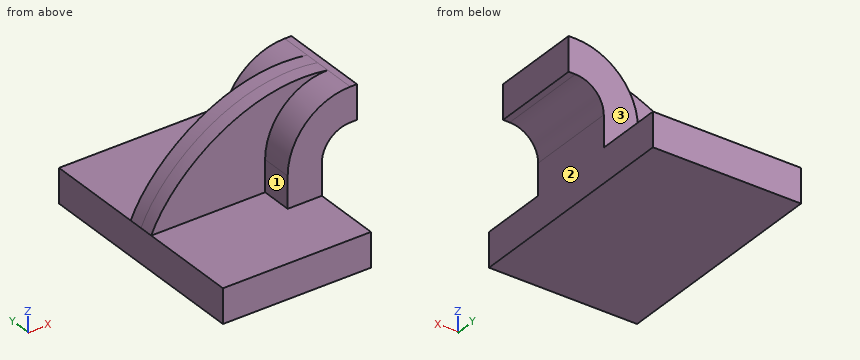
```python
from build123d import *

# Parameters (mm, degrees)
F1_DEPTH = 63.5
F2_DEPTH = 25.4
F3_DEPTH = 7.9375


with BuildPart() as f1:
    # F0 (on Front) → F1 (new body, symmetric)
    with BuildSketch(Plane.XZ):
        Polygon((-41.275, 9.525), (-41.275, -9.525), (41.275, -9.525), (41.275, 9.525), (22.225, 9.525), align=None)
    extrude(amount=F1_DEPTH, both=True)

    # F0 (on Front) → F2 (join, symmetric)
    with BuildSketch(Plane.XZ):
        with BuildLine():
            Line((22.225, 9.525), (41.275, 9.525))
            Line((41.275, 9.525), (41.275, 27.0002))
            ThreePointArc((41.275, 27.0002), (45.9246798487, 38.2255201513), (57.15, 42.8752))
            Line((57.15, 42.8752), (60.8642640084, 42.8752))
            Line((60.8642640084, 42.8752), (60.8642640084, 61.9252))
            Line((60.8642640084, 61.9252), (57.15, 61.9252))
            ThreePointArc((57.15, 61.9252), (32.4542956671, 51.6959043329), (22.225, 27.0002))
            Line((22.225, 27.0002), (22.225, 9.525))
        make_face()
    extrude(amount=F2_DEPTH, both=True)

    # F0 (on Front) → F3 (join, symmetric)
    with BuildSketch(Plane.XZ):
        with BuildLine():
            add(Edge.make_bspline(
                [(-41.275, 9.525), (-30.5388011038, 34.9970385432), (9.5851859078, 69.7711631656), (57.15, 61.9252)],
                knots=[0, 0, 0, 0, 111.5045361635, 111.5045361635, 111.5045361635, 111.5045361635], degree=3))
            Line((-41.275, 9.525), (22.225, 9.525))
            Line((22.225, 9.525), (22.225, 27.0002))
            ThreePointArc((22.225, 27.0002), (32.4542956671, 51.6959043329), (57.15, 61.9252))
        make_face()
    extrude(amount=F3_DEPTH, both=True)


solid = f1.part
```
CAD build for the part. Positions are in the model's coordinates, mm. Face numbers are marked on the shaded views. A direction names the side the tool comes from. Give positions to 0.01 mm unless a question says otherwise; leave off trailing zeros. Order: outer loops, then holes, each group sorted by start corner. A loop starts at its lowest first (then second) coordinate and runs counter-clockwise, first axis right, second up. Notation, with made-up numbers: M 53.25,67.25 L 103.25,67.25 A21 cw 103.25,94.25 Z; hole C 30,43 d7. An arc over 180 degrees is marked long. Put each result on its own line as item: value. Start each with the question number.
(1) Which spindle directions (+Z, -Z, +X, -X, +Y, -Y) get a long thin tool onto all of the face, cutting with end or side? Do the marked faces 1, 2 and 3. Say none if no direction does.
(2) Flat gauge pins, fed straight in: pin 1 Ø1.9 at (x, y) = (59, -9.5) entering from -Z; pin 2 Ø1.9 at (x, y) = (59, -9.5) entering from +Z; pin 3 Ø5 at (y, z) = (14, 19) entering from +X (3 decimals). Where does each tip first touch, or does it go through?
(3) Drill centre lines: line 1 along Y through (x, z) = (-25, 14.5); line 2 along Z through (x, y) = (-31, 27.5) (3 decimals); line 3 along X through (y, z) = (12, 8.5) (3 decimals). Where is each one in solid material? Low to high.
(4) Saw through at A-A, the plane y = -49.5. Write the cut outline in (x, z) (3 decimals).
Check result:
1. face 1: +Z, -X, -Y
1. face 2: -Z, +X, +Y, -Y
1. face 3: +Z, +X, -X, +Y
2. pin 1: stops at z = 42.88
2. pin 2: stops at z = 61.93
2. pin 3: stops at x = 41.275
3. line 1: y = -7.94 to 7.94
3. line 2: z = -9.525 to 9.525
3. line 3: x = -41.275 to 41.275
4. outline: M -41.275,-9.525 L 41.275,-9.525 L 41.275,9.525 L -41.275,9.525 Z
